CAD build for the part. Positions are in the model's coordinates, mm. Face numbers are marked on the shaded views. Give positions to 0.01 mm unless a question says otherwise; leave off trailing zeros. Order: outer loops, then holes, each group sorted by start corner. A loop starts at its lowest first (then second) coordinate and runs counter-clockwise, first axis right, second up. Notation, with made-up numbers: (10, 57) -> (56, 57) arc R25 cw to (56, 89) -> close; hole circle Ø9 at (-31.75, 29). An arc over 180 degrees is marked (long way). Answer as CSV lines item,"result".
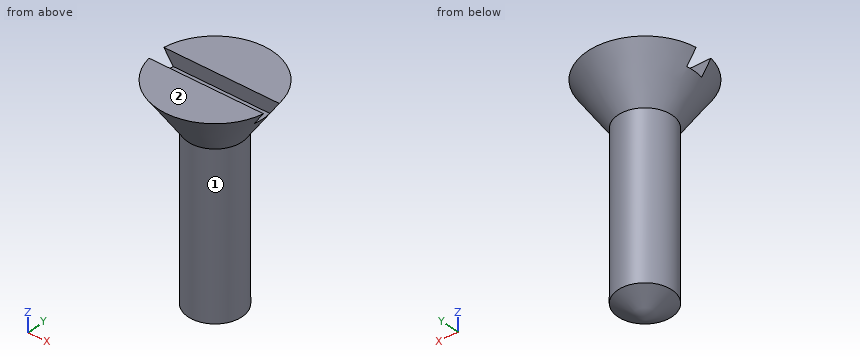
Autodesk Inventor part; units mm, degrees
ref_plane "YZ Plane" through (0, 0, 0) normal (1, 0, 0) x (0, 1, 0)
ref_plane "XZ Plane" through (0, 0, 0) normal (0, 1, 0) x (-1, 0, 0)
ref_plane "XY Plane" through (0, 0, 0) normal (0, 0, 1) x (1, 0, 0)
sketch "Sketch3" plane through (0, 0, 0) normal (0, 0, 1) x (1, 0, 0)
  circle A0 centre (0, 0) radius 3
  dimension "d9" = 6
extrude "Extrusion1" add sketch "Sketch3" against normal blind 18
sketch "Sketch4" plane through (0, 0, 0) normal (1, 0, 0) x (0, 1, 0)
  line L0 (-3, -18) -> (3, -18)
  line L1 (0, -19.7321) -> (3, -18)
  line L2 (0, -18) -> (0, -19.7321)
  point P0 (0, 0)
revolve "Revolution1" add sketch "Sketch4" angle 360 mid plane about axis through (0, 0, -18) along (0, 0, -1)
sketch "Sketch5" plane through (0, 0, 0) normal (0, 1, 0) x (-1, 0, 0)
  line L0 (3, 0) -> (-3, 0)
  line L1 (3, 0) -> (6.385, 5)
  line L2 (6.385, 5) -> (0, 5)
  line L3 (0, 5) -> (0, 0)
  dimension "d14" = 5
  dimension "d15" = 6.385
revolve "Revolution2" add sketch "Sketch5" angle 360 about axis through (0, 0, 5) along (0, 0, -1)
sketch "Sketch6" plane through (0, 0, 0) normal (1, 0, 0) x (0, 1, 0)
  line L0 (-6.385, 5) -> (6.385, 5)
  line L1 (-1.15, 5) -> (-1.15, 3.5)
  line L2 (-1.15, 3.5) -> (-0.15, 3.5)
  line L3 (-0.15, 3.5) -> (0.85, 3.5)
  line L4 (0.85, 3.5) -> (0.85, 5)
  point P0 (0, 0)
  dimension "d17" = 1
  dimension "d18" = 1.5
extrude "Extrusion2" cut sketch "Sketch6" along normal mid plane 20
properties part number "Pieza7_tornillo" material "Iron, Cast"
1) Pin check, flat tips, straight feed: P1, Ø3, axis at y = 0.5, z = -10, coming from the +X side; P2, Ø1.5, axis at y = -5, z = -2, coming from the -X side; P3, Ø1.2, axis at x = 1.5, z = 4.5, coming from the +Y side; P4, Ø1, axis at x = 0.5, y = 2, coming from the -Z side. Stop position of each tip, or through.
Data:
P1,"stops at x = 3"
P2,"passes through"
P3,"stops at y = 6.28"
P4,"stops at z = -18.83"
2) Wall check: line 1 along X through (y, z) = (0, -17.75); line 2 along Z through (x, y) = (0.25, 4.75); line 3 along X through (y, z) = (0, 2.75). Give the ranges that are in metal, low to high. Write a range as [from, to].
Data:
line 1,"x = [-3, 3]"
line 2,"z = [2.59, 5]"
line 3,"x = [-4.86, 4.86]"
3) Band-saw the part on A-A, the plane z = 0.5. Write the cut outline in (x, y).
Data:
outline,"circle Ø6.68 at (0, 0)"
4) Band-saw the part on B-B, the plane z = -8.75. Write the cut outline in (x, y), then the cut area to 3 significant figures.
Data:
outline,"circle Ø6 at (0, 0)"
area,"28.3 mm2"
5) Pull direction Y, two halves, no side cores. Call the marked faces 1 and 2: pulls with the +Y half, pulls with the -Y half, needs draft (parallel to the pull), parting line crosses it, or undercut.
Data:
face 1,"parting line crosses it"
face 2,"needs draft"
